```python
from build123d import *

# Parameters (mm, degrees)
SKETCH1_W           = 138
SKETCH1_H           = 42
BOSS_EXTRUDE1_DEPTH = 28
BOSS_EXTRUDE2_START = -14
BOSS_EXTRUDE2_DEPTH = 105


with BuildPart() as part:
    # Sketch1 → Boss-Extrude1 (new body)
    with BuildSketch(Plane(origin=(0, 0, 0), x_dir=(1, 0, 0), z_dir=(0, 1, 0))):
        Rectangle(SKETCH1_W, SKETCH1_H)
    extrude(amount=BOSS_EXTRUDE1_DEPTH)

    # Sketch3 → Boss-Extrude2 (add)
    with BuildSketch(Plane(origin=(69, 0, 0), x_dir=(0, 0, -1), z_dir=(1, 0, 0)).offset(BOSS_EXTRUDE2_START)):
        Polygon((-15, -5), (15, -5), (10, 0), (-10, 0), align=None)
    extrude(amount=-BOSS_EXTRUDE2_DEPTH)


solid = part.part
```
Work out the finished part from the listing and answer in its coordinate system (mm). A direction names the side the tool comes from. Give positions to 0.01 mm unless a question says otherwise; leave off trailing zeros. Order: outer loops, then holes, each group sorted by start corner. A loop starts at its lowest first (then second) coordinate and runs counter-clockwise, first axis right, second up.
1. Section A-A, the plane z = 6 is taken. Determine the outline of the cut face in (x, y).
Result sheet:
outline: (-69, 0) - (-50, 0) - (-50, -5) - (55, -5) - (55, 0) - (69, 0) - (69, 28) - (-69, 28) - close
2. This flat-tipped pin is pushed along its axis until it touches: P1, Ø1.5, axis at y = -1.5, z = -4.5, coming from the -X side. Where does it stop, or does it pass through?
Result sheet:
P1: stops at x = -50
3. Section B-B, the plane x = -35.5 is taken. Determine the outline of the cut face in (y, z).
Result sheet:
outline: (-5, -15) - (0, -10) - (0, -21) - (28, -21) - (28, 21) - (0, 21) - (0, 10) - (-5, 15) - close
4. The mould has two halves that part along Y. Classify faces 1 (the flat face through (-50, -2, 0)), 2 (the flat face through (-1, 28, 0)), 3 (the flat face through (3, -3, -13)), 4 (the flat face through (3, -2, 12)): released by +Y, released by -Y, zero draft, split by the parting line, or undercut.
Result sheet:
face 1: zero draft
face 2: released by +Y
face 3: undercut
face 4: undercut
5. For faces 5 (the flat face through (3, -5, 0)), 6 (the flat face through (55, -2, 0)), determine the directions among +Z, -Z, +X, -X, +Y, -Y from which every point of the face is accessible in a straight line to the end or side of a thin tool.
Result sheet:
face 5: +Z, -Z, +X, -X, -Y
face 6: +Z, -Z, +X, -Y
6. Straight lines are drawn through the part: L1, parallel to Y at x = 53.5, z = -15.5; L2, parallel to Y at x = -0.5, z = 13.5; L3, parallel to Y at x = 18, z = 12.5. For each, find the intervals that lie inside material, in ascending order.
Result sheet:
L1: y = 0 to 28
L2: y = -5 to -3.5, 0 to 28
L3: y = -5 to -2.5, 0 to 28
